Design review of the part built by this model. Coordinates are the model's own, in mm. Face numbers are marked on the shaded views. A direction names the side the tool comes from. Give positions to 0.01 mm unless a question says otherwise; leave off trailing zeros. Loops run counter-clockwise (first coordinate to the right, second up) from the corner with the lowest first, then second, coordinate; pieces in that order, holes last. Notation, with made-up numbers: (24.25, 6.25) - (55.25, 6.25) arc R8 ccw to (55.25, 16.25) - close; hole circle Ø5 at (-10, -27). An arc over 180 degrees is marked (long way). Write each question's results on one line, items separated by ' | '.
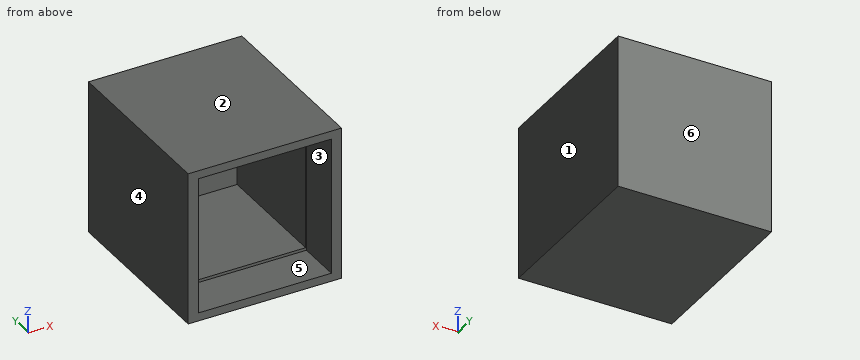
```python
from build123d import *

# Parameters (mm, degrees)
SKETCH1_W           = 140
SKETCH1_H           = 160
SKETCH1_W_2         = 120
SKETCH1_H_2         = 140
EXTRUDE_THIN1_DEPTH = 60
SKETCH2_W           = 140
SKETCH2_H           = 160
BOSS_EXTRUDE1_DEPTH = 10
SKETCH5_W           = 140
SKETCH5_H           = 160
BOSS_EXTRUDE2_DEPTH = 10
SKETCH7_W           = 121.54877743
SKETCH7_H           = 125.094770936
CUT_EXTRUDE2_DEPTH  = 40


with BuildPart() as part:
    # Sketch1 → Extrude-Thin1 (new, symmetric)
    with BuildSketch(Plane.XY):
        Rectangle(SKETCH1_W, SKETCH1_H)
        Rectangle(SKETCH1_W_2, SKETCH1_H_2, mode=Mode.SUBTRACT)
    extrude(amount=EXTRUDE_THIN1_DEPTH, both=True)

    # Sketch2 → Boss-Extrude1 (add)
    with BuildSketch(Plane.XY.offset(60)):
        Rectangle(SKETCH2_W, SKETCH2_H)
    extrude(amount=BOSS_EXTRUDE1_DEPTH)

    # Sketch5 → Boss-Extrude2 (add)
    with BuildSketch(Plane(origin=(0, 0, -60), x_dir=(-1, 0, 0), z_dir=(0, 0, -1))):
        Rectangle(SKETCH5_W, SKETCH5_H)
    extrude(amount=BOSS_EXTRUDE2_DEPTH)

    # Sketch7 → Cut-Extrude2 (cut)
    with BuildSketch(Plane.XZ.offset(80)):
        Rectangle(SKETCH7_W, SKETCH7_H)
    extrude(amount=-CUT_EXTRUDE2_DEPTH, mode=Mode.SUBTRACT)


solid = part.part
```
Item 1: Draft analysis for pull direction X (two halves, no side actions). For the marked faces 1, 2, 3 and 4, state which applies: +X half, -X half, draft (parallel to the pull), parting line (faces both ways), or undercut.
Output values:
face 1: +X half | face 2: draft | face 3: undercut | face 4: -X half
Item 2: We need section B-B on z = 27.5. Give the boundary of the cut face in (x, y).
Output values:
outline: (-70, -80) - (-60.77, -80) - (-60.77, -40) - (-60, -40) - (-60, 70) - (60, 70) - (60, -40) - (60.77, -40) - (60.77, -80) - (70, -80) - (70, 80) - (-70, 80) - close
Item 3: We need section D-D on y = -43. Give the boundary of the cut face in (x, z).
Output values:
outline: (-70, -70) - (70, -70) - (70, 70) - (-70, 70) - close; hole (-60.77, -62.55) - (60.77, -62.55) - (60.77, 62.55) - (-60.77, 62.55) - close
Item 4: We need section C-C on x = -42. Give the boundary of the cut face in (y, z), then the cut area to 3 significant figures.
Output values:
outline: (-80, -70) - (80, -70) - (80, 70) - (-80, 70) - (-80, 62.55) - (-40, 62.55) - (-40, 60) - (70, 60) - (70, -60) - (-40, -60) - (-40, -62.55) - (-80, -62.55) - close | area: 4,200 mm²
Item 5: Wall thickness on probe 1 along X at (y, z) = (-26.5, -21.5); probe 2 along X at (y, z) = (-57.5, 60): over which ranges is each line inside the solid? List them lowest first.
Output values:
probe 1: x = -70 to -60, 60 to 70 | probe 2: x = -70 to -60.77, 60.77 to 70
Item 6: Tool access review of the marked faces 5 and 6: name each direction out of +Z, -Z, +X, -X, +Y, -Y from which nothing blocks a thin tool from reaching the whole face with its end or side.
Output values:
face 5: -Y | face 6: +Z, -Z, +X, -X, +Y
Item 7: We need section A-A on y = 14. Give the boundary of the cut face in (x, z).
Output values:
outline: (-70, -70) - (70, -70) - (70, 70) - (-70, 70) - close; hole (-60, -60) - (60, -60) - (60, 60) - (-60, 60) - close
Item 8: Clearance check with a flat-ended pin moving along its axis: P1, Ø1, axis at x = -53, z = -41, coming from the -Y side. State where the tip first meets the part, or that it passes through.
Output values:
P1: stops at y = 70
